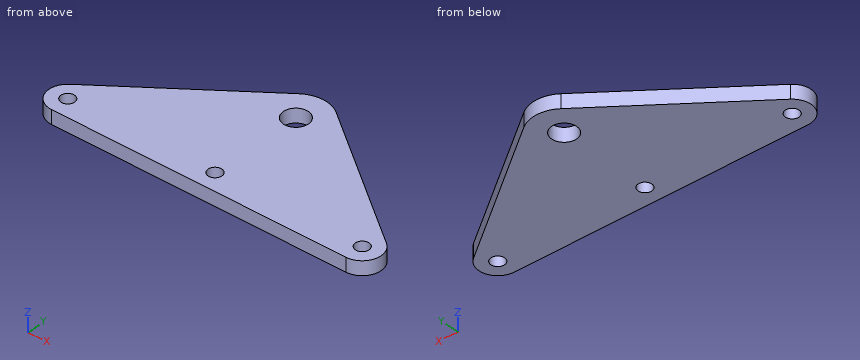
Autodesk Inventor part; units mm, degrees
ref_plane "YZ Plane" through (0, 0, 0) normal (1, 0, 0) x (0, 1, 0)
ref_plane "XZ Plane" through (0, 0, 0) normal (0, 1, 0) x (-1, 0, 0)
ref_plane "XY Plane" through (0, 0, 0) normal (0, 0, 1) x (1, 0, 0)
sketch "Sketch1" plane through (0, 0, 0) normal (0, 0, 1) x (1, 0, 0)
  circle A0 centre (0, 0) radius 20
  circle A1 centre (-235, -150) radius 11
  circle A2 centre (0, -150) radius 11
  arc A3 (-252.9136, -125.9354) -> (-235, -180) centre (-235, -150) ccw
  line L0 (0, 87.1559) -> (0, -290.9336) construction
  circle A4 centre (235, -150) radius 11
  arc A5 (235, -180) -> (252.9136, -125.9354) centre (235, -150) ccw
  line L1 (-235, -180) -> (235, -180)
  arc A6 (29.8559, 40.1076) -> (-29.8559, 40.1076) centre (0, 0) ccw
  line L2 (-252.9136, -125.9354) -> (-29.8559, 40.1076)
  line L3 (252.9136, -125.9354) -> (29.8559, 40.1076)
  point P0 (0, -180)
  point P1 (0, 46.2314)
  dimension "d0" = 40
  dimension "d1" = 22
  dimension "d3" = 22
  dimension "d4" = 150
  dimension "d8" = 235
  dimension "d16" = 470
  dimension "d17" = 30
  dimension "d18" = 100
extrude "Extrusion1" add sketch "Sketch1" along normal mid plane 22.22
equation "\"d1\" = d3"
properties part number "Corpo_Suporte_3_Cabos_Modelo1"
The model under review builds one solid part; all positions refer to its coordinate system, in mm. Round coordinates to 2 decimals unless told otherwise and drop trailing zeros. Order: outer loops, then holes, each group sorted by start corner. A loop starts at its lowest first (then second) coordinate and runs counter-clockwise, first axis right, second up.
(1) Take a section at D-D, the plane y = 10. State the section outline as (x, z) points, plus the area to 3 significant figures.
Working result:
outline: (-70.3, -11.11) - (-17.32, -11.11) - (-17.32, 11.11) - (-70.3, 11.11) - close; (17.32, -11.11) - (70.3, -11.11) - (70.3, 11.11) - (17.32, 11.11) - close
area: 2,350 mm2
(2) For P1, Ø6, axis at x = 186, z = 1, coming from the +Y side; P2, Ø10, axis at y = -20.5, z = 3.5, coming from the +X side; P3, Ø10, axis at y = -38, z = -6.5, coming from the -X side, all flat-tipped, find the tip position at first contact; note any pin that passes through.
Working result:
P1: stops at y = -73.89
P2: stops at x = 117.99
P3: stops at x = -141.5
(3) Wall thickness on L1, parallel to Y at x = -227.5, z = -7.25; L2, parallel to Y at x = 235, z = -6.5; L3, parallel to X at y = 11, z = 3: over which ranges is each line inside the solid? List them lowest first.
Working result:
L1: y = -180 to -158.05, -141.95 to -107.02
L2: y = -180 to -161, -139 to -112.6
L3: x = -68.96 to -16.7, 16.7 to 68.96
(4) Take a section at B-B, the plane y = -150. State the section outline as (x, z) points.
Working result:
outline: (-265, -11.11) - (-246, -11.11) - (-246, 11.11) - (-265, 11.11) - close; (-224, -11.11) - (-11, -11.11) - (-11, 11.11) - (-224, 11.11) - close; (11, -11.11) - (224, -11.11) - (224, 11.11) - (11, 11.11) - close; (246, -11.11) - (265, -11.11) - (265, 11.11) - (246, 11.11) - close
(5) Take a section at A-A, the plane x = 0. State the section outline as (y, z) points.
Working result:
outline: (-180, -11.11) - (-161, -11.11) - (-161, 11.11) - (-180, 11.11) - close; (-139, -11.11) - (-20, -11.11) - (-20, 11.11) - (-139, 11.11) - close; (20, -11.11) - (50, -11.11) - (50, 11.11) - (20, 11.11) - close
(6) Take a section at C-C, the plane z = 7. State the section outline as (x, y) points, plus the area to 4 significant figures.
Working result:
outline: (-252.91, -125.94) arc R30 ccw to (-235, -180) - (235, -180) arc R30 ccw to (252.91, -125.94) - (29.86, 40.11) arc R50 ccw to (-29.86, 40.11) - close; hole circle Ø22 at (-235, -150); hole circle Ø40 at (0, 0); hole circle Ø22 at (0, -150); hole circle Ø22 at (235, -150)
area: 73,050 mm2
